Geometry check sheet. Reference: the model listing, model coordinates, mm. Give positions to 0.01 mm unless a question says otherwise; leave off trailing zeros. Loops run counter-clockwise (first coordinate to the right, second up) from the corner with the lowest first, then second, coordinate; pieces in that order, holes last. Notation, with made-up numbers: (-38.5, 27.5) -> (9.5, 27.5) arc R19 ccw to (9.5, 42.5) -> close; hole circle Ø2 at (71.5, -27). An arc over 180 degrees is marked (long way). Answer as a JSON object with one key per item and string values.
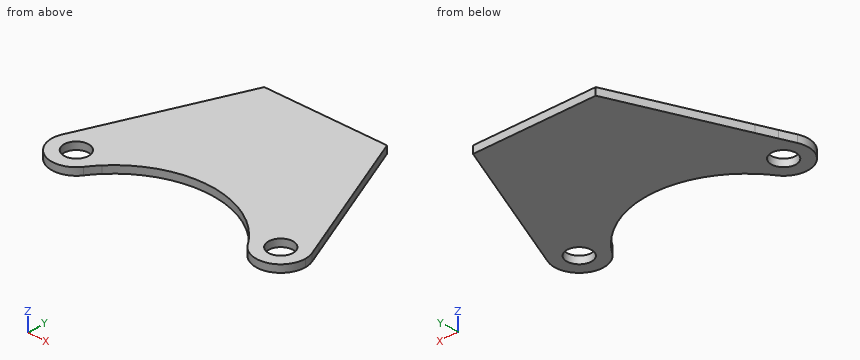
from build123d import *

# Parameters (mm, degrees)
F0_R     = 10
F1_DEPTH = 6


with BuildPart() as f1:
    # F0 (on Top) → F1 (new body)
    with BuildSketch(Plane.XY):
        with BuildLine():
            ThreePointArc((66.8107155763, 68.8983527146), (89.2220086446, 61.1485010982), (103.2801650714, 80.2454771665))
            ThreePointArc((103.2801650714, 80.2454771665), (102.8817929615, 84.2174016446), (101.7025466654, 88.0310957293))
            ThreePointArc((101.7025466654, 88.0310957293), (73.6640874011, 97.7820404055), (66.8107155763, 68.8983527146))
        make_face()
        with Locations((83.2801650714, 80.2454771665)):
            Circle(F0_R, mode=Mode.SUBTRACT)
        with BuildLine():
            ThreePointArc((66.8107155763, 68.8983527146), (73.6640874011, 97.7820404055), (101.7025466654, 88.0310957293))
            Line((101.7025466654, 88.0310957293), (96.8992238213, 99.3967496769))
            ThreePointArc((96.8992238213, 99.3967496769), (71.3236564608, 100.476441104), (59.9351524158, 77.550967172))
            ThreePointArc((59.9351524158, 77.550967172), (63.5204352748, 73.3418677958), (66.8107155763, 68.8983527146))
        make_face()
        with BuildLine():
            ThreePointArc((59.9351524158, 77.550967172), (71.3236564608, 100.476441104), (96.8992238213, 99.3967496769))
            Line((96.8992238213, 99.3967496769), (90.8352022654, 113.7454771665))
            Line((90.8352022654, 113.7454771665), (-90.8352022654, 113.7454771665))
            Line((-90.8352022654, 113.7454771665), (-96.8992238213, 99.3967496769))
            ThreePointArc((-96.8992238213, 99.3967496769), (-72.5051449003, 101.1296563534), (-59.7801650714, 80.2454771665))
            ThreePointArc((-59.7801650714, 80.2454771665), (-59.8189439032, 78.8959953041), (-59.9351524158, 77.550967172))
            ThreePointArc((-59.9351524158, 77.550967172), (0, 104), (59.9351524158, 77.550967172))
        make_face()
        with BuildLine():
            ThreePointArc((-66.8107155763, 68.8983527146), (-63.5204352748, 73.3418677958), (-59.9351524158, 77.550967172))
            ThreePointArc((-59.9351524158, 77.550967172), (-59.8189439032, 78.8959953041), (-59.7801650714, 80.2454771665))
            ThreePointArc((-59.7801650714, 80.2454771665), (-72.5051449003, 101.1296563534), (-96.8992238213, 99.3967496769))
            Line((-96.8992238213, 99.3967496769), (-101.7025466654, 88.0310957293))
            ThreePointArc((-101.7025466654, 88.0310957293), (-79.3082405933, 99.8471050565), (-63.2801650714, 80.2454771665))
            ThreePointArc((-63.2801650714, 80.2454771665), (-64.1831890032, 74.3036335933), (-66.8107155763, 68.8983527146))
        make_face()
        with BuildLine():
            ThreePointArc((-101.7025466654, 88.0310957293), (-92.8962427418, 62.7089139274), (-66.8107155763, 68.8983527146))
            ThreePointArc((-66.8107155763, 68.8983527146), (-64.1831890032, 74.3036335933), (-63.2801650714, 80.2454771665))
            ThreePointArc((-63.2801650714, 80.2454771665), (-79.3082405933, 99.8471050565), (-101.7025466654, 88.0310957293))
        make_face()
        with Locations((-83.2801650714, 80.2454771665)):
            Circle(F0_R, mode=Mode.SUBTRACT)
        Polygon((-90.8352022654, 113.7454771665), (90.8352022654, 113.7454771665), (50, 210.37), (0, 210.37), (-50, 210.37), align=None)
    extrude(amount=F1_DEPTH)


solid = f1.part
1) Section check C-C on y = 130. Record the cut outline in (x, z).
Geometry check:
{"outline": "(-83.97, 0) -> (83.97, 0) -> (83.97, 6) -> (-83.97, 6) -> close"}
2) Section check D-D on x = -1.5. Record the cut outline in (y, z), plus the area to 3 significant figures.
Geometry check:
{"outline": "(103.99, 0) -> (210.37, 0) -> (210.37, 6) -> (103.99, 6) -> close", "area": "638 mm2"}
3) Depth check by flat-ended pin: P1, Ø18, axis at x = -83.28, y = 80.25, coming from the +Z side; P2, Ø2, axis at x = -32.5, z = 4, coming from the -Y side; P3, Ø3, axis at y = 96.5, z = 4.5, coming from the +X side. Enter the tip coordinate at first touch or a pass-through.
Geometry check:
{"P1": "passes through", "P2": "stops at y = 96.76", "P3": "stops at x = 98.76"}
4) Material ranges on line 1 along X through (y, z) = (86, 1.85); line 2 along X through (y, z) = (71, 3.6); line 3 along Y through (x, z) = (-89.5, 1.3), recorded low to high. Write a range as from..to.
Geometry check:
{"line 1": "x = -102.43..-91.46, -75.1..-50.96, 50.96..75.1, 91.46..102.43", "line 2": "x = -101.01..-87.09, -79.47..-65.31, 65.31..79.47, 87.09..101.01", "line 3": "y = 61.24..72.42, 88.08..116.9"}
5) Section check A-A on z = 4. Record the cut outline in (x, y).
Geometry check:
{"outline": "(-101.7, 88.03) arc R20 ccw to (-66.81, 68.9) arc R81.13 cw to (66.81, 68.9) arc R20 ccw to (101.7, 88.03) -> (50, 210.37) -> (-50, 210.37) -> close; hole circle Ø20 at (-83.28, 80.25); hole circle Ø20 at (83.28, 80.25)"}
6) Section check B-B on x = 78. Record the cut outline in (y, z).
Geometry check:
{"outline": "(60.96, 0) -> (71.75, 0) -> (71.75, 6) -> (60.96, 6) -> close; (88.74, 0) -> (144.12, 0) -> (144.12, 6) -> (88.74, 6) -> close"}
